```python
from build123d import *

# Parameters (mm, degrees)
F1_DEPTH = 1.2
F3_DEPTH = 7.5
F5_DEPTH = 1.2
F6_R     = 0.59999


# Not quite as in the source:
# - a fillet or chamfer is up to 0.001 mm smaller than in the source, because OpenCascade refuses the exact size


with BuildPart() as f1:
    # F0 (on Front) → F1 (new body)
    with BuildSketch(Plane.XZ):
        Polygon((-28.9807687655, 0), (-30.1807687655, 0), (-30.1807687655, -40), (24.3192312345, -40), (24.3192312345, 0), (23.1192312345, 0), (23.1192312345, -38.8), (-28.9807687655, -38.8), align=None)
        Polygon((-2.9307687655, -19.4), (-28.9807687655, 0), (-28.9807687655, -38.8), align=None)
        with BuildLine():
            Line((23.1192312345, 0), (-28.9807687655, 0))
            Line((-28.9807687655, 0), (-2.9307687655, -19.4))
            Line((-2.9307687655, -19.4), (-2.9307687655, -11.2695819765))
            ThreePointArc((-2.9307687655, -11.2695819765), (-3.9914289373, -8.7089218048), (-1.4307687655, -9.7695819765))
            Line((-1.4307687655, -9.7695819765), (3.4249790478, -9.7695819765))
            Line((3.4249790478, -9.7695819765), (3.4249790478, -14.6667367532))
            Line((3.4249790478, -14.6667367532), (23.1192312345, 0))
        make_face()
        Polygon((23.1192312345, -38.8), (23.1192312345, 0), (3.4249790478, -14.6667367532), (3.4249790478, -19.4), (3.3088028431, -19.4), (3.3088028431, -24.0467443074), align=None)
        with BuildLine():
            Line((-2.9307687655, -19.4), (-28.9807687655, -38.8))
            Line((-28.9807687655, -38.8), (23.1192312345, -38.8))
            Line((23.1192312345, -38.8), (3.3088028431, -24.0467443074))
            Line((3.3088028431, -24.0467443074), (3.3088028431, -29.0304180235))
            Line((3.3088028431, -29.0304180235), (-1.4307687655, -29.0304180235))
            ThreePointArc((-1.4307687655, -29.0304180235), (-3.9914289373, -30.0910781952), (-2.9307687655, -27.5304180235))
            Line((-2.9307687655, -27.5304180235), (-2.9307687655, -19.4))
        make_face()
        with BuildLine():
            Line((3.3088028431, -24.0467443074), (-2.9307687655, -19.4))
            Line((-2.9307687655, -19.4), (-2.9307687655, -27.5304180235))
            ThreePointArc((-2.9307687655, -27.5304180235), (-1.8701085937, -27.9697578517), (-1.4307687655, -29.0304180235))
            Line((-1.4307687655, -29.0304180235), (3.3088028431, -29.0304180235))
            Line((3.3088028431, -29.0304180235), (3.3088028431, -24.0467443074))
        make_face()
        Polygon((3.3088028431, -19.4), (-2.9307687655, -19.4), (3.3088028431, -24.0467443074), align=None)
        Polygon((3.4249790478, -14.6667367532), (-2.9307687655, -19.4), (3.3088028431, -19.4), (3.4249790478, -19.4), align=None)
        with BuildLine():
            Line((-2.9307687655, -11.2695819765), (-2.9307687655, -19.4))
            Line((-2.9307687655, -19.4), (3.4249790478, -14.6667367532))
            Line((3.4249790478, -14.6667367532), (3.4249790478, -9.7695819765))
            Line((3.4249790478, -9.7695819765), (-1.4307687655, -9.7695819765))
            ThreePointArc((-1.4307687655, -9.7695819765), (-1.8701085937, -10.8302421483), (-2.9307687655, -11.2695819765))
        make_face()
    extrude(amount=F1_DEPTH)

    # F2 (on face) → F3 (join)
    with BuildSketch(Plane.XZ.offset(1.2)):
        Polygon((-30.1807687655, 0), (-30.1807687655, -40), (24.3192312345, -40), (24.3192312345, 0), (23.1192312345, 0), (23.1192312345, -38.8), (-28.9807687655, -38.8), (-28.9807687655, 0), align=None)
    extrude(amount=F3_DEPTH)

    # F4 (on face) → F5 (join)
    with BuildSketch(Plane.XZ.offset(8.7)):
        with BuildLine():
            Line((-25.1807687655, 0), (-28.9807687655, 0))
            Line((-28.9807687655, 0), (-28.9807687655, -38.8))
            Line((-28.9807687655, -38.8), (23.1192312345, -38.8))
            Line((23.1192312345, -38.8), (23.1192312345, 0))
            Line((23.1192312345, 0), (19.3192312345, 0))
            Line((19.3192312345, 0), (19.3192312345, -26))
            ThreePointArc((19.3192312345, -26), (18.7334447969, -27.4142135624), (17.3192312345, -28))
            Line((17.3192312345, -28), (-23.1807687655, -28))
            ThreePointArc((-23.1807687655, -28), (-24.5949823279, -27.4142135624), (-25.1807687655, -26))
            Line((-25.1807687655, -26), (-25.1807687655, 0))
        make_face()
        Polygon((-30.1807687655, 0), (-30.1807687655, -40), (24.3192312345, -40), (24.3192312345, 0), (23.1192312345, 0), (23.1192312345, -38.8), (-28.9807687655, -38.8), (-28.9807687655, 0), align=None)
    extrude(amount=F5_DEPTH)

    # F6 (radius 0.6 in the source; OpenCascade refuses exactly that, so slightly less here)
    f6_edges = [f1.edges().sort_by_distance(p)[0] for p in [
        (-30.180769, -4.95, -40),
        (24.319231, -4.95, -40),
        (-30.180769, -4.95, 0),
        (-27.680769, -9.9, 0),
        (24.319231, -4.95, 0),
        (21.819231, -9.9, 0),
        (-2.930769, -9.9, -40),
        (24.319231, -9.9, -20),
        (-30.180769, -9.9, -20),
        (-25.180769, -9.9, -13),
        (-2.930769, -8.7, -28),
        (19.319231, -8.7, -13),
        (-27.080769, -8.7, 0),
        (-28.980769, -4.95, 0),
        (23.119231, -4.95, 0),
        (21.219231, -8.7, 0),
        (19.319231, -9.3, 0),
        (-25.180769, -9.3, 0),
        (-2.930769, -1.2, 0),
    ]]
    fillet(f6_edges, radius=F6_R)


solid = f1.part
```
Geometry check sheet. Reference: the model listing, model coordinates, mm. A direction names the side the tool comes from. Give positions to 0.01 mm unless a question says otherwise; leave off trailing zeros. Loops run counter-clockwise (first coordinate to the right, second up) from the corner with the lowest first, then second, coordinate; pieces in that order, holes last. Notation, with made-up numbers: (-8, -5) - (29, -5) arc R22 ccw to (29, 23) - close; hole circle Ø6 at (59.25, 24). An arc over 180 degrees is marked (long way). Use CSV: the item, a comma, the result in double quotes. Start each with the question number.
Q1. Section check C-C, the plane z = -35.5. Record the cut outline in (x, y), and give its area (3 significant figures).
Q2. Release check for a two-part mould opening along X. For faces 3 (the face through (-3, -5, -38.8)), 4 (the face through (-3, -5, -40)), 5 (the face through (-30.181, -5, -20)) record: +X half, -X half, draft (parallel to the pull), parting line (faces both ways), or undercut.
Q3. Access from +Z, -Z, +X, -X, +Y, -Y to the whole of each face (thin tool, end or side, straight path). Record for faces 1 (the face through (-2.8, -0.2, 0)), 2 (the face through (-3, -1.2, -19)).
Q4. Scan lines: probe 1 along X at (y, z) = (-7.5, -17.5); probe 2 along Y at (x, z) = (-23, -38); probe 3 along Y at (x, z) = (-8, -18). Record each from-to range of solid material in increasing order. Write a range as from..to.
Q5. Go/stop test with flat-tipped pins: pin 1 Ø5 at (x, z) = (-22, -21) entering from -Y; pin 2 Ø2 at (x, y) = (2, -6.5) entering from +Z. Record where each tip stops, or that it passes through.
Findings below:
1,outline,"(-30.18, -9.3) arc R0.6 ccw to (-29.58, -9.9) - (23.72, -9.9) arc R0.6 ccw to (24.32, -9.3) - (24.32, 0) - (-30.18, 0) - close; hole (-28.98, -8.7) - (23.12, -8.7) - (23.12, -1.2) - (-28.98, -1.2) - close"
1,area,"149 mm^2"
2,face 3,"undercut"
2,face 4,"draft"
2,face 5,"-X half"
3,face 1,"+Z, +X, -X, +Y, -Y"
3,face 2,"+Z"
4,probe 1,"x = -30.18..-28.98, 23.12..24.32"
4,probe 2,"y = -9.9..-8.7, -1.2..0"
4,probe 3,"y = -1.2..0"
5,pin 1,"stops at y = -1.2"
5,pin 2,"stops at z = -38.8"
